from build123d import *

# Parameters (mm, degrees)
F0_R           = 0.79375
F1_DEPTH       = 25.4
F3_START       = -1.5875
F2_R           = 1.93675
F3_DEPTH       = 1.5875
F5_START       = 1.5875
F4_R           = 1.93675
F5_DEPTH       = 1.5875
F7_START       = 1.5875
F6_R           = 1.93675
F7_DEPTH       = 1.5875
F9_START       = 1.5875
F8_R           = 1.93675
F9_DEPTH       = 1.5875
F11_START      = 1.5875
F10_R          = 1.93675
F11_DEPTH      = 1.5875
F13_START      = 1.5875
F12_R          = 1.93675
F13_DEPTH      = 1.5875
F14_R          = 0.79375
F15_DEPTH      = 23.8135
F16_R          = 0.79375
F17_DEPTH      = 23.8135
F19_DEPTH      = 25.4
F19_DEPTH_BACK = 25.4
F20_R          = 3.175
F21_DEPTH      = 25.4


with BuildPart() as f1:
    # F0 (on Front) → F1 (new body)
    with BuildSketch(Plane.XZ):
        with BuildLine():
            ThreePointArc((1.5896937253, 0.4764627531), (2.6960840616, -0.0482905293), (3.7380205176, -0.6915898416))
            Line((3.7380205176, -0.6915898416), (3.7380205176, 1.9999169571))
            Line((3.7380205176, 1.9999169571), (-0.6752294824, 1.9999169571))
            Line((-0.6752294824, 1.9999169571), (-1.2424904239, 1.4326560155))
            ThreePointArc((-1.2424904239, 1.4326560155), (-1.1342950237, 1.3151450731), (-1.0361511327, 1.1891179217))
            ThreePointArc((-1.0361511327, 1.1891179217), (-0.0353529614, 0.9985724567), (0.9437888558, 0.7171726424))
            ThreePointArc((0.9437888558, 0.7171726424), (1.336612932, 0.7843066024), (1.5896937253, 0.4764627531))
        make_face()
        with BuildLine():
            ThreePointArc((-0.6752294824, 0.0631669571), (-0.7905484204, -0.5951562531), (-1.1227724786, -1.1750830429))
            Line((-1.1227724786, -1.1750830429), (3.7380205176, -1.1750830429))
            Line((3.7380205176, -1.1750830429), (3.7380205176, -0.6915898416))
            ThreePointArc((3.7380205176, -0.6915898416), (2.6960840616, -0.0482905293), (1.5896937253, 0.4764627531))
            ThreePointArc((1.5896937253, 0.4764627531), (1.5935929319, 0.4445453037), (1.5948955176, 0.4124169571))
            ThreePointArc((1.5948955176, 0.4124169571), (1.0297772788, 0.0529674082), (0.9437888558, 0.7171726424))
            ThreePointArc((0.9437888558, 0.7171726424), (-0.0353529614, 0.9985724567), (-1.0361511327, 1.1891179217))
            ThreePointArc((-1.0361511327, 1.1891179217), (-0.7676657728, 0.654358553), (-0.6752294824, 0.0631669571))
        make_face()
        with BuildLine():
            ThreePointArc((-2.6119794826, -1.8735830429), (3.0006805932, -4.1984229672), (5.3255205176, -9.8110830429))
            ThreePointArc((5.3255205176, -9.8110830429), (3.0006805933, -15.4237431186), (-2.6119794824, -17.7485830429))
            ThreePointArc((-2.6119794824, -17.7485830429), (-1.7895380331, -17.9318819815), (-1.1227724786, -18.4470830429))
            Line((-1.1227724786, -18.4470830429), (0.6491882277, -18.4470830429))
            ThreePointArc((0.6491882277, -18.4470830429), (1.8330205176, -17.3834580429), (3.0168528075, -18.4470830429))
            Line((3.0168528075, -18.4470830429), (3.7380205176, -18.4470830429))
            Line((3.7380205176, -18.4470830429), (3.7380205176, -18.9305762443))
            ThreePointArc((3.7380205176, -18.9305762443), (3.777174424, -18.9031877834), (3.8162102016, -18.8756312191))
            ThreePointArc((3.8162102016, -18.8756312191), (5.7845599908, -18.2076225161), (6.4525686938, -16.2392727269))
            ThreePointArc((6.4525686938, -16.2392727269), (6.4801252581, -16.2002369493), (6.507513719, -16.1610830429))
            Line((6.507513719, -16.1610830429), (6.0240205176, -16.1610830429))
            Line((6.0240205176, -16.1610830429), (6.0240205176, -3.4610830429))
            Line((6.0240205176, -3.4610830429), (6.507513719, -3.4610830429))
            ThreePointArc((6.507513719, -3.4610830429), (6.4801252581, -3.4219291366), (6.4525686938, -3.382893359))
            ThreePointArc((6.4525686938, -3.382893359), (5.7845599908, -1.4145435697), (3.8162102016, -0.7465348668))
            ThreePointArc((3.8162102016, -0.7465348668), (3.777174424, -0.7189783025), (3.7380205176, -0.6915898416))
            Line((3.7380205176, -0.6915898416), (3.7380205176, -1.1750830429))
            Line((3.7380205176, -1.1750830429), (-1.1227724786, -1.1750830429))
            ThreePointArc((-1.1227724786, -1.1750830429), (-1.7895380332, -1.6902841045), (-2.6119794826, -1.8735830429))
        make_face()
        with Locations((4.1232126084, -16.5462751337)):
            Circle(F0_R, mode=Mode.SUBTRACT)
        with Locations((4.1232126084, -3.0758909521)):
            Circle(F0_R, mode=Mode.SUBTRACT)
        with BuildLine():
            Line((0.6491882277, -18.4470830429), (-1.1227724786, -18.4470830429))
            ThreePointArc((-1.1227724786, -18.4470830429), (-0.7905484204, -19.0270098328), (-0.6752294824, -19.6853330429))
            ThreePointArc((-0.6752294824, -19.6853330429), (-0.7676657728, -20.2765246389), (-1.0361511327, -20.8112840076))
            ThreePointArc((-1.0361511327, -20.8112840076), (1.4609745046, -20.150265896), (3.7380205176, -18.9305762443))
            Line((3.7380205176, -18.9305762443), (3.7380205176, -18.4470830429))
            Line((3.7380205176, -18.4470830429), (3.0168528075, -18.4470830429))
            ThreePointArc((3.0168528075, -18.4470830429), (3.0219461273, -18.5104922792), (3.0236455176, -18.5740830429))
            ThreePointArc((3.0236455176, -18.5740830429), (1.7694297539, -19.7630086526), (0.6491882277, -18.4470830429))
        make_face()
        with BuildLine():
            ThreePointArc((3.7380205176, -18.9305762443), (1.4609745046, -20.150265896), (-1.0361511327, -20.8112840076))
            ThreePointArc((-1.0361511327, -20.8112840076), (-1.7258883381, -21.4074953601), (-2.6119794824, -21.6220830429))
            Line((-2.6119794824, -21.6220830429), (3.7380205176, -21.6220830429))
            Line((3.7380205176, -21.6220830429), (3.7380205176, -18.9305762443))
        make_face()
    extrude(amount=-F1_DEPTH)

    # F2 (on face) → F3 (join)
    with BuildSketch(Plane(origin=(0, 25.4, 0), x_dir=(-1, 0, 0), z_dir=(0, 1, 0)).offset(F3_START)):
        with Locations((2.6119794824, 0.0631669571)):
            Circle(F2_R)
        with Locations((2.6119794824, -19.6853330429)):
            Circle(F2_R)
    extrude(amount=-F3_DEPTH)

    # F4 (on face) → F5 (join)
    with BuildSketch(Plane.XZ.offset(-22.225).offset(F5_START)):
        with Locations((-2.6119794824, 0.0631669571)):
            Circle(F4_R)
    extrude(amount=F5_DEPTH)

    # F6 (on face) → F7 (join)
    with BuildSketch(Plane.XZ.offset(-19.05).offset(F7_START)):
        with Locations((-2.6119794824, 0.0631669571)):
            Circle(F6_R)
    extrude(amount=F7_DEPTH)

    # F8 (on face) → F9 (join)
    with BuildSketch(Plane.XZ.offset(-15.875).offset(F9_START)):
        with Locations((-2.6119794824, 0.0631669571)):
            Circle(F8_R)
    extrude(amount=F9_DEPTH)

    # F10 (on face) → F11 (join)
    with BuildSketch(Plane.XZ.offset(-12.7).offset(F11_START)):
        with Locations((-2.6119794824, 0.0631669571)):
            Circle(F10_R)
    extrude(amount=F11_DEPTH)

    # F12 (on face) → F13 (join)
    with BuildSketch(Plane.XZ.offset(-22.225).offset(F13_START)):
        with Locations((-2.6119794824, -19.6853330429)):
            Circle(F12_R)
    extrude(amount=F13_DEPTH)

    # F14 (on face) → F15 (cut, through all)
    with BuildSketch(Plane(origin=(0, 23.8125, 0), x_dir=(-1, 0, 0), z_dir=(0, 1, 0))):
        with Locations((2.6119794824, 0.0631669571)):
            Circle(F14_R)
    extrude(amount=-F15_DEPTH, mode=Mode.SUBTRACT)

    # F16 (on face) → F17 (cut, through all)
    with BuildSketch(Plane(origin=(0, 23.8125, 0), x_dir=(-1, 0, 0), z_dir=(0, 1, 0))):
        with Locations((2.6119794824, -19.6853330429)):
            Circle(F16_R)
    extrude(amount=-F17_DEPTH, mode=Mode.SUBTRACT)

    # F18 (on face) → F19 (cut, two sides)
    with BuildSketch(Plane.YZ.offset(6.0240205176)) as f19_sk:
        Polygon((21.9337120652, -25.8094575256), (25.4, -21.6220830429), (15.4893942562, -9.8110830429), (15.4893942562, 6.843551062), (-6.1063589528, 6.843551062), (-6.1063589528, -25.8094575256), align=None)
    extrude(amount=-F19_DEPTH, mode=Mode.SUBTRACT)
    extrude(f19_sk.sketch, amount=F19_DEPTH_BACK, mode=Mode.SUBTRACT)

    # F20 (on face) → F21 (cut)
    with BuildSketch(Plane.YZ.offset(6.0240205176)):
        with Locations((15.4893942562, -9.8110830429)):
            Circle(F20_R)
    extrude(amount=-F21_DEPTH, mode=Mode.SUBTRACT)


solid = f1.part
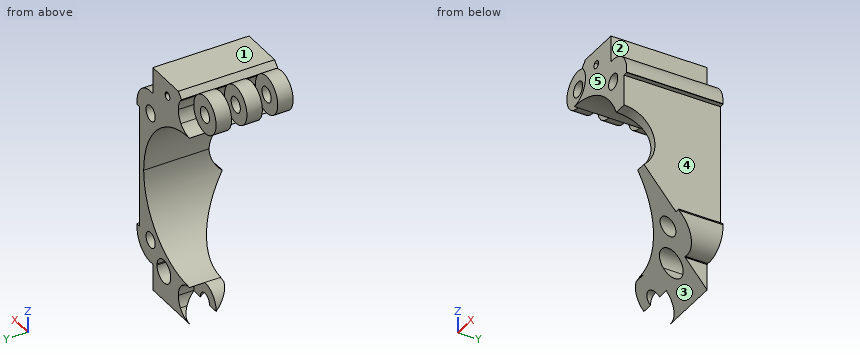
Source: CAD feature listing. Evaluate the final solid. Frame: model axes, mm. Face numbers are marked on the shaded views. A direction names the side the tool comes from. Give positions to 0.01 mm unless a question says otherwise; leave off trailing zeros. Order: outer loops, then holes, each group sorted by start corner. A loop starts at its lowest first (then second) coordinate and runs counter-clockwise, first axis right, second up. Notation, with made-up numbers: (30, 64) -> (85, 64) arc R17 ccw to (85, 69) -> close; hole circle Ø2 at (29.5, -1). An arc over 180 degrees is marked (long way). Write item = value, one per line.
Q1. Material intervals for line 1 (X direction, y = 23.75, z = -9.75); line 2 (Z direction, x = 1, y = 18.75); line 3 (Z direction, x = 2, y = 21.5), sorted ascending. Write a range as from..to.
Data:
line_1 = 5.33..6.02
line_2 = -2.74..0.07, 0.76..2
line_3 = -16.97..-16.27, -3.35..2
Q2. Set-up query: the marked faces 1 and 2. Return all of +Z, -Z, +X, -X, +Y, -Y with unobstructed straight access to the full face (end or side cutting, diameter ignored); none if empty.
Data:
face_1 = +Z, +X, -X, +Y, -Y
face_2 = +Z, +X, +Y, -Y
Q3. Pull-direction query (Z, two-part tool) for the marked faces 3, 4 and 5; classes: released by +Z, released by -Z, zero draft, split by the parting line, or undercut.
Data:
face_3 = released by -Z
face_4 = undercut
face_5 = zero draft
Q4. Pin query (flat end, axial travel): pin 1 (3 mm diameter, centred on x = -2.5, z = 0, fed in from +Y); pin 2 (1.3 mm diameter, centred on x = -2.61, z = 0.06, fed in from -Y); pin 3 (3 mm diameter, centred on y = 19.5, z = 0, fed in from +X); pin 4 (3 mm diameter, centred on y = 22.5, z = -18.5, fed in from -X). Return the tip coordinate at first contact, or that it passes through.
Data:
pin_1 = 23.81
pin_2 = through
pin_3 = 5.87
pin_4 = -4.54
Q5. Cut plane B-B, the plane x = 0.25. Output: boundary loops of the cut face in (y, z), and give its area (3 significant figures).
Data:
outline = (15.49, -2.41) -> (25.4, -2.41) -> (25.4, 2) -> (15.49, 2) -> close; (21.7, -17.21) -> (25.4, -21.62) -> (25.4, -17.21) -> close
area = 51.8 mm^2
Q6. Cut plane A-A, the plane y = 18.25. State how many separate pieces and enclosed holes the cut face has, and give its area (3 significant figures).
Data:
separate_pieces = 2
enclosed_holes = 2
area = 38.3 mm^2
